For this review, take the finished solid that the model builds, in its own axes (mm). A direction names the side the tool comes from. Round coordinates to 2 decimals unless told otherwise and drop trailing zeros. Write each loop counter-clockwise with the first axis right and the second up, starting at its lowest first coordinate (ties: lowest second). Pieces come first, ordered by that corner, then holes. Notation, with made-up numbers: (40, -29.5) -> (76, -29.5) arc R29 cw to (76, -2.5) -> close; hole circle Ø8 at (18, 28.5). An arc over 180 degrees is marked (long way). Answer in a Markdown table with one row per item.
from build123d import *

# Parameters (mm, degrees)
BOSS_EXTRUDE1_DEPTH = 45
SKETCH2_R           = 1.25
BOSS_EXTRUDE2_DEPTH = 7
FILLET1_R           = 8
BOSS_EXTRUDE3_DEPTH = 8.5
SKETCH7_W           = 12
SKETCH7_H           = 9.5
CUT_EXTRUDE1_DEPTH  = 7
BOSS_EXTRUDE4_DEPTH = 10
SKETCH9_W           = 3.98
SKETCH9_H           = 1.98
BOSS_EXTRUDE5_DEPTH = 2.98
SKETCH11_W          = 31.5
SKETCH11_H          = 9.530048311
BOSS_EXTRUDE6_DEPTH = 7
SKETCH16_R          = 1
BOSS_EXTRUDE7_DEPTH = 10
FILLET2_R           = 1
FILLET4_R           = 0.5
FILLET5_R           = 0.5
FILLET6_R           = 0.5
FILLET7_R           = 8
FILLET8_DEPTH       = 18.5
FILLET8_START       = 18.5
FILLET8_2_DEPTH     = 26.5
SKETCH17_R          = 8
CUT_EXTRUDE2_DEPTH  = 57.192438403
SKETCH18_W          = 26.905399266
SKETCH18_H          = 5.924124609
CUT_EXTRUDE3_DEPTH  = 5
SKETCH19_W          = 27.645914842
SKETCH19_H          = 7.775413549
CUT_EXTRUDE4_DEPTH  = 5


with BuildPart() as part:
    # Sketch1 → Boss-Extrude1 (new body)
    with BuildSketch(Plane.XY):
        Polygon((-6.049640288, 0), (-0.949640288, 0), (-0.949640288, -2.9), (-7.849640288, -2.9), (-7.849640288, 5.1), (12.150359712, 5.1), (12.150359712, -2.9), (5.250359712, -2.9), (5.250359712, 0), (10.350359712, 0), (10.350359712, 2.6), (-6.049640288, 2.6), align=None)
    extrude(amount=BOSS_EXTRUDE1_DEPTH)

    # Sketch2 → Boss-Extrude2 (add)
    with BuildSketch(Plane.XY.offset(45)):
        Polygon((-19.349640288, 25.6), (-19.349640288, 5.1), (12.650359712, 5.1), (12.650359712, 25.6), (7.650359712, 25.6), (7.650359712, 14.6), (-14.349640288, 14.6), (-14.349640288, 25.6), align=None)
        with Locations((10.150359712, 20.1)):
            Circle(SKETCH2_R, mode=Mode.SUBTRACT)
        with Locations((-16.849640288, 20.1)):
            Circle(SKETCH2_R, mode=Mode.SUBTRACT)
    extrude(amount=-BOSS_EXTRUDE2_DEPTH)

    # Fillet1
    # the kernel refuses this fillet: 8 mm, written as the material it adds along each edge
    with BuildSketch(Plane(origin=(-7.849640288, 5.1, 38), x_dir=(0, -1, 0), z_dir=(0, 0, 1))) as fillet1_piece_1:
        with BuildLine():
            CenterArc((FILLET1_R, -FILLET1_R), FILLET1_R, 90, 90)
            Line((0, -FILLET1_R), (0, 0))
            Line((0, 0), (FILLET1_R, 0))
        make_face()
    extrude(amount=7)
    with BuildSketch(Plane(origin=(12.150359712, 5.1, 38), x_dir=(0, -1, 0), z_dir=(0, 0, 1))) as fillet1_piece_2:
        with BuildLine():
            CenterArc((2.783882181, 8), FILLET1_R, 249.635865194, 20.364134806)
            Line((0, 0.5), (0, 0))
            Line((0, 0), (2.783882181, 0))
        make_face()
    extrude(amount=7)

    # Sketch4 → Boss-Extrude3 (add)
    with BuildSketch(Plane(origin=(0, 0, 0), x_dir=(-1, 0, 0), z_dir=(0, 0, -1))):
        Polygon((-18.150359712, 15.6), (-18.150359712, 5.1), (13.849640288, 5.1), (13.849640288, 15.6), (5.349640288, 15.6), (5.349640288, 26.6), (-9.650359712, 26.6), (-9.650359712, 15.6), align=None)
    extrude(amount=-BOSS_EXTRUDE3_DEPTH)

    # Sketch7 → Cut-Extrude1 (cut)
    with BuildSketch(Plane.XY.offset(8.5)):
        with Locations((0.650359712, 20.35)):
            Rectangle(SKETCH7_W, SKETCH7_H)
    extrude(amount=-CUT_EXTRUDE1_DEPTH, mode=Mode.SUBTRACT)

    # Sketch8 → Boss-Extrude4 (add)
    with BuildSketch(Plane.XY.offset(8.5)):
        with BuildLine():
            Line((-13.849640288, 15.6), (-12.158728309, 15.6))
            ThreePointArc((-12.158728309, 15.6), (2.150359712, 5.1), (16.459447733, 15.6))
            Line((16.459447733, 15.6), (18.150359712, 15.6))
            Line((18.150359712, 15.6), (18.150359712, 3.937972429))
            Line((18.150359712, 3.937972429), (-13.849640288, 3.937972429))
            Line((-13.849640288, 3.937972429), (-13.849640288, 15.6))
        make_face()
    extrude(amount=BOSS_EXTRUDE4_DEPTH)

    # Sketch9 → Boss-Extrude5 (add)
    with BuildSketch(Plane.XY.offset(8.5)):
        with Locations((2.150359712, 13.1)):
            Rectangle(SKETCH9_W, SKETCH9_H)
    extrude(amount=BOSS_EXTRUDE5_DEPTH)

    # Sketch11 → Boss-Extrude6 (add)
    with BuildSketch(Plane(origin=(0, 0, 38), x_dir=(-1, 0, 0), z_dir=(0, 0, -1))):
        with Locations((3.599640288, 9.865024156)):
            Rectangle(SKETCH11_W, SKETCH11_H)
    extrude(amount=BOSS_EXTRUDE6_DEPTH)

    # Sketch16 → Boss-Extrude7 (add)
    # profile 1 of 2: a face of its own
    with BuildSketch(Plane.XY.offset(18.5)):
        with BuildLine():
            Line((-13.346805139, 15.601949196), (-13.846805139, 15.601949196))
            Line((-13.846805139, 15.601949196), (-13.849640288, 14.1))
            Line((-13.849640288, 14.1), (-14.815015575, 15.247623037))
            ThreePointArc((-14.815015575, 15.247623037), (-15.7608574, 17.911832315), (-13.346805139, 16.44044538))
            Line((-13.346805139, 16.44044538), (-13.346805139, 15.601949196))
        make_face()
        with Locations((-14.815015575, 16.747623037)):
            Circle(SKETCH16_R, mode=Mode.SUBTRACT)
    # profile 2 of 2: a face of its own
    with BuildSketch(Plane.XY.offset(18.5)):
        with BuildLine():
            Line((17.652000257, 15.6), (18.150359712, 15.6))
            Line((18.150359712, 15.6), (18.150359712, 14.1))
            Line((18.150359712, 14.1), (19.116258964, 15.247623037))
            ThreePointArc((19.116258964, 15.247623037), (20.054810716, 17.91771731), (17.652000257, 16.422128892))
            Line((17.652000257, 16.422128892), (17.652000257, 15.6))
        make_face()
        with Locations((19.116258964, 16.747623037)):
            Circle(SKETCH16_R, mode=Mode.SUBTRACT)
    extrude(amount=-BOSS_EXTRUDE7_DEPTH)

    # Fillet2
    fillet2_edges = [part.edges().sort_by_distance(p)[0] for p in [
        (-13.849640288, 14.1, 13.5),
        (-14.815015575, 15.247623037, 13.5),
        (19.116258964, 15.247623037, 13.5),
        (18.150359712, 14.1, 13.5),
    ]]
    fillet(fillet2_edges, radius=FILLET2_R)

    # Fillet4
    fillet4_edges = [part.edges().sort_by_distance(p)[0] for p in [
        (0.160359712, 13.1, 11.48),
        (2.150359712, 12.11, 11.48),
        (4.140359712, 13.1, 11.48),
        (2.150359712, 14.09, 11.48),
    ]]
    fillet(fillet4_edges, radius=FILLET4_R)

    # Fillet5
    fillet5_edges = [part.edges().sort_by_distance(p)[0] for p in [
        (6.650359712, 20.35, 8.5),
        (0.650359712, 25.1, 8.5),
    ]]
    fillet(fillet5_edges, radius=FILLET5_R)

    # Fillet6
    fillet6_edges = [part.edges().sort_by_distance(p)[0] for p in [
        (-14.349640288, 20.115024155, 38),
        (7.650359712, 20.115024155, 38),
    ]]
    fillet(fillet6_edges, radius=FILLET6_R)

    # Fillet7
    fillet7_edges = [part.edges().sort_by_distance(p)[0] for p in [
        (-7.849640288, 5.1, 34.5),
    ]]
    fillet(fillet7_edges, radius=FILLET7_R - 0.0001)  # a hair under: the kernel refuses the full size

    # Fillet8: read off the stored shape, not the designer's step
    # Fillet8 outline → Fillet8 (add)
    with BuildSketch(Plane.XY):
        with BuildLine():
            Line((18.150359712, 5.1), (12.150359712, 5.1))
            Line((12.150359712, 5.1), (12.150359712, -2.645966692))
            ThreePointArc((12.150359712, -2.645966692), (13.825804392, 2.253012793), (18.150359712, 5.1))
        make_face()
        with BuildLine():
            Line((-7.849640288, 5.1), (-13.849640288, 5.1))
            ThreePointArc((-13.849640288, 5.1), (-9.525084967, 2.253012794), (-7.849640288, -2.645966692))
            Line((-7.849640288, -2.645966692), (-7.849640288, 5.1))
        make_face()
    extrude(amount=FILLET8_DEPTH)

    # Fillet8 2 outline → Fillet8 2 (add)
    with BuildSketch(Plane.XY.offset(FILLET8_START)):
        with BuildLine():
            Line((-7.849640288, 5.1), (-13.849640288, 5.1))
            ThreePointArc((-13.849640288, 5.1), (-9.525084967, 2.253012794), (-7.849640288, -2.645966692))
            Line((-7.849640288, -2.645966692), (-7.849640288, 5.1))
        make_face()
    extrude(amount=FILLET8_2_DEPTH)

    # Sketch17 → Cut-Extrude2 (cut, through all)
    with BuildSketch(Plane.XY.offset(45)):
        with Locations((-15.895053234, -2.569483857)):
            Circle(SKETCH17_R)
        with Locations((20.210973801, -2.569483857)):
            Circle(SKETCH17_R)
    extrude(amount=-CUT_EXTRUDE2_DEPTH, mode=Mode.SUBTRACT)

    # Sketch18 → Cut-Extrude3 (cut)
    with BuildSketch(Plane.XY.offset(45)):
        with Locations((1.903783169, -0.265657621)):
            Rectangle(SKETCH18_W, SKETCH18_H)
    extrude(amount=-CUT_EXTRUDE3_DEPTH, mode=Mode.SUBTRACT)

    # Sketch19 → Cut-Extrude4 (cut)
    with BuildSketch(Plane(origin=(0, 0, 0), x_dir=(-1, 0, 0), z_dir=(0, 0, -1))):
        with Locations((-1.944922923, -1.314721353)):
            Rectangle(SKETCH19_W, SKETCH19_H)
    extrude(amount=-CUT_EXTRUDE4_DEPTH, mode=Mode.SUBTRACT)


solid = part.part
1) For faces 4 (the flat face through (9.65, 21, 4)), 5 (the flat face through (12, 2.573, 2)), 6 (the flat face through (5.25, -1, 22)), 7 (the flat face through (4.14, 13, 10)), list the 3-axis set-ups (+Z, -Z, +X, -X, +Y, -Y) from which the entire face can be reached by the end or side of a thin tool; tool diameter is ignored.
Solved:
| item | result |
|---|---|
| face 4 | -Z, +X, +Y |
| face 5 | -Z, +X, -X, -Y |
| face 6 | +Z, -Z, -Y |
| face 7 | +Y |
2) Clearance check with flat-ended pins moving along their axes: pin 1 Ø3 at (x, y) = (-16.85, 20.1) entering from +Z; pin 2 Ø1.8 at (x, y) = (-14.82, 16.75) entering from -Z; pin 3 Ø12 at (x, z) = (-7.5, 16) entering from +Y; pin 4 Ø8 at (x, z) = (-13.5, 33.5) entering from +Y. State where each tip first meets the part, or that it passes through.
Solved:
| item | result |
|---|---|
| pin 1 | z = 45 |
| pin 2 | z = 38 |
| pin 3 | y = 17.47 |
| pin 4 | y = 14.63 |
3) Mouldability with a two-part tool opening along Z and no side actions: class faces 1 (the flat face through (-6.05, 1, 24)), 2 (the flat face through (0.16, 13, 10)), 3 (the flat face through (11.4, 19, 38)) as pulls with the +Z half, pulls with the -Z half, needs draft (parallel to the pull), parting line crosses it, or undercut.
Solved:
| item | result |
|---|---|
| face 1 | needs draft |
| face 2 | undercut |
| face 3 | undercut |
4) Consider section B-B on z = 29.5. State the section outline as (x, y) points.
Solved:
| item | result |
|---|---|
| outline | (-13.62, 5.1) arc R8 cw to (-8.99, 1.48) arc R8 cw to (-7.85, -2.65) -> (-7.85, -2.9) -> (-0.95, -2.9) -> (-0.95, 0) -> (-6.05, 0) -> (-6.05, 2.6) -> (10.35, 2.6) -> (10.35, 0) -> (5.25, 0) -> (5.25, -2.9) -> (12.15, -2.9) -> (12.15, 5.1) -> close |
5) Consider section A-A on y = 23. State the section outline as (x, z) points, then the cut area to 3 significant figures.
Solved:
| item | result |
|---|---|
| outline | (-19.35, 38) -> (-14.85, 38) arc R0.5 ccw to (-14.35, 38.5) -> (-14.35, 45) -> (-19.35, 45) -> close; (-5.35, 0) -> (9.65, 0) -> (9.65, 8.5) -> (7.15, 8.5) arc R0.5 ccw to (6.65, 8) -> (6.65, 1.5) -> (-5.35, 1.5) -> close; (7.65, 38.5) arc R0.5 ccw to (8.15, 38) -> (12.65, 38) -> (12.65, 45) -> (7.65, 45) -> close |
| area | 113 mm² |
6) Consider section C-C on z = 41. State the section outline as (x, y) points, then the cut area to 3 significant figures.
Solved:
| item | result |
|---|---|
| outline | (-19.35, 5.1) -> (-18.17, 5.1) arc R8 cw to (-9.87, 2.7) -> (12.16, 2.7) arc R8 cw to (12.65, 5.1) -> (12.65, 25.6) -> (7.65, 25.6) -> (7.65, 14.6) -> (-14.35, 14.6) -> (-14.35, 25.6) -> (-19.35, 25.6) -> close; hole circle Ø2.5 at (-16.85, 20.1); hole circle Ø2.5 at (10.15, 20.1) |
| area | 460 mm² |
7) For line 1 (Z direction, x = -6, y = 11.5); line 2 (Z direction, x = 6.5, y = 22.25); line 3 (Y direction, x = 11, z = 6), list the stretches that pass through material, from the lowest coordinate up. Write a range as [from, to].
Solved:
| item | result |
|---|---|
| line 1 | [0, 8.5], [31, 45] |
| line 2 | [0, 1.5] |
| line 3 | [-2.9, 15.6] |
8) Consider section D-D on y = 7. State the section outline as (x, z) points, then the cut area to 3 significant figures.
Solved:
| item | result |
|---|---|
| outline | (-19.35, 31) -> (12.15, 31) -> (12.15, 38) -> (12.65, 38) -> (12.65, 45) -> (-19.35, 45) -> close; (-13.85, 0) -> (18.15, 0) -> (18.15, 18.5) -> (9.46, 18.5) -> (9.46, 8.5) -> (-5.16, 8.5) -> (-5.16, 18.5) -> (-13.85, 18.5) -> close |
| area | 890 mm² |
